```python
from build123d import *

# Parameters (mm, degrees)
SKETCH1_R               = 6.35
BOSS_EXTRUDE1_DEPTH     = 5.08
SKETCH2_R               = 6.35
SKETCH2_R_2             = 1.143
BOSS_EXTRUDE2_DEPTH     = 3.175
TAP_DRILL_FOR_M3_TAP2_D = 2.5


with BuildPart() as part:
    # Sketch1 → Boss-Extrude1 (new body)
    with BuildSketch(Plane.XY):
        Circle(SKETCH1_R)
        with BuildLine():
            Line((-2.413, -2.54), (-2.413, 2.54))
            ThreePointArc((-2.413, 2.54), (0, 3.503451013), (2.413, 2.54))
            Line((2.413, 2.54), (2.413, -2.54))
            ThreePointArc((2.413, -2.54), (0, -3.503451013), (-2.413, -2.54))
        make_face(mode=Mode.SUBTRACT)
    extrude(amount=BOSS_EXTRUDE1_DEPTH)

    # Sketch2 → Boss-Extrude2 (add)
    with BuildSketch(Plane.XY.offset(5.08)):
        Circle(SKETCH2_R)
        Circle(SKETCH2_R_2, mode=Mode.SUBTRACT)
    extrude(amount=BOSS_EXTRUDE2_DEPTH)

    # Tap Drill for M3 Tap2 (through all)
    with Locations(Plane(origin=(0, 0, 0), x_dir=(-1, 0, 0), z_dir=(0, 0, -1))):
        with Locations((-4.699, 0), (4.699, 0)):
            Hole(TAP_DRILL_FOR_M3_TAP2_D / 2)


solid = part.part
```
CAD build for the part. Positions are in the model's coordinates, mm. A direction names the side the tool comes from. Give positions to 0.01 mm unless a question says otherwise; leave off trailing zeros. Write each loop counter-clockwise with the first axis right and the second up, starting at its lowest first coordinate (ties: lowest second). Pieces come first, ordered by that corner, then holes. Notation, with made-up numbers: M -21,-4 L -3,-4 A11 ccw -3,2 Z; hole C 39,31 d1. An arc over 180 degrees is marked long. Return JSON: item names as keys, results as strings. Group by question number.
(1) 3-axis set-ups, long thin cutter, end or side, ignore diameter. For faces 4 (the face through (1.3, 0.1, 8.255)), 5 (the face through (-2.413, 0, 3)): which of +Z, -Z, +X, -X, +Y, -Y reach the whole face in a straight line?
(2) Mould opens along Y. For faces 1 (the face through (3, 0, 0)), 2 (the face through (-0.037, 3.503, 2.504)), 3 (the face through (-1.38, -6.2, 4.07)) say: pulls with the +Y half, pulls with the -Y half, needs draft (parallel to the pull), parting line crosses it, or undercut.
(3) Flat gauge pins, fed straight in: pin 1 Ø1.5 at (y, z) = (-1, 2) entering from +X; pin 2 Ø2 at (x, y) = (4.699, 0) entering from -Z; pin 3 Ø1.5 at (x, z) = (2.5, 3) entering from +Y; pin 4 Ø3 at (y, z) = (3, 3) entering from -X. Where does each tip first touch, or does it go through?
(4) Drill centre lines: L1, parallel to Y at x = 5, z = 7.5; L2, parallel to X at y = -2, z = 1; L3, parallel to Y at x = -4.75, z = 7.75. Where is each one in solid material? Low to high. Write a range as [from, to].
(5) Band-saw the part on A-A (y = 0). Give the cut face in (x, z) (3 decimals).
(6) Band-saw the part on D-D (y = -3). Give the cut face in (x, z) (3 decimals).
(7) Band-saw the part on B-B (z = 4.25). Give the cut face in (x, y), and give its area (3 significant figures).
(8) Band-saw the part on C-C (x = 0). Give the cut face in (y, z) (3 decimals), and give its area (3 significant figures).
Entries:
{
 "1": {"face 4": "+Z, +X, -X, +Y, -Y", "face 5": "-Z"},
 "2": {"face 1": "needs draft", "face 2": "undercut", "face 3": "parting line crosses it"},
 "3": {"pin 1": "stops at x = 6.35", "pin 2": "passes through", "pin 3": "stops at y = 6.1", "pin 4": "stops at x = -6.17"},
 "4": {"L1": "y = [-3.91, -1.21], [1.21, 3.91]", "L2": "x = [-6.03, -2.41], [2.41, 6.03]", "L3": "y = [-4.21, -1.25], [1.25, 4.21]"},
 "5": {"outline": "M -6.35,0 L -5.949,0 L -5.949,8.255 L -6.35,8.255 Z; M -3.449,0 L -2.413,0 L -2.413,5.08 L -1.143,5.08 L -1.143,8.255 L -3.449,8.255 Z; M 1.143,5.08 L 2.413,5.08 L 2.413,0 L 3.449,0 L 3.449,8.255 L 1.143,8.255 Z; M 5.949,0 L 6.35,0 L 6.35,8.255 L 5.949,8.255 Z"},
 "6": {"outline": "M -5.597,0 L -1.809,0 L -1.809,5.08 L 1.809,5.08 L 1.809,0 L 5.597,0 L 5.597,8.255 L -5.597,8.255 Z"},
 "7": {"outline": "C 0,0 d12.7; hole C -4.7,0 d2.5; hole M -2.41,-2.54 A3.5 ccw 2.41,-2.54 L 2.41,2.54 A3.5 ccw -2.41,2.54 Z; hole C 4.7,0 d2.5", "area": "86.0 mm^2"},
 "8": {"outline": "M -6.35,0 L -3.503,0 L -3.503,5.08 L -1.143,5.08 L -1.143,8.255 L -6.35,8.255 Z; M 1.143,5.08 L 3.503,5.08 L 3.503,0 L 6.35,0 L 6.35,8.255 L 1.143,8.255 Z", "area": "62.0 mm^2"}
}
